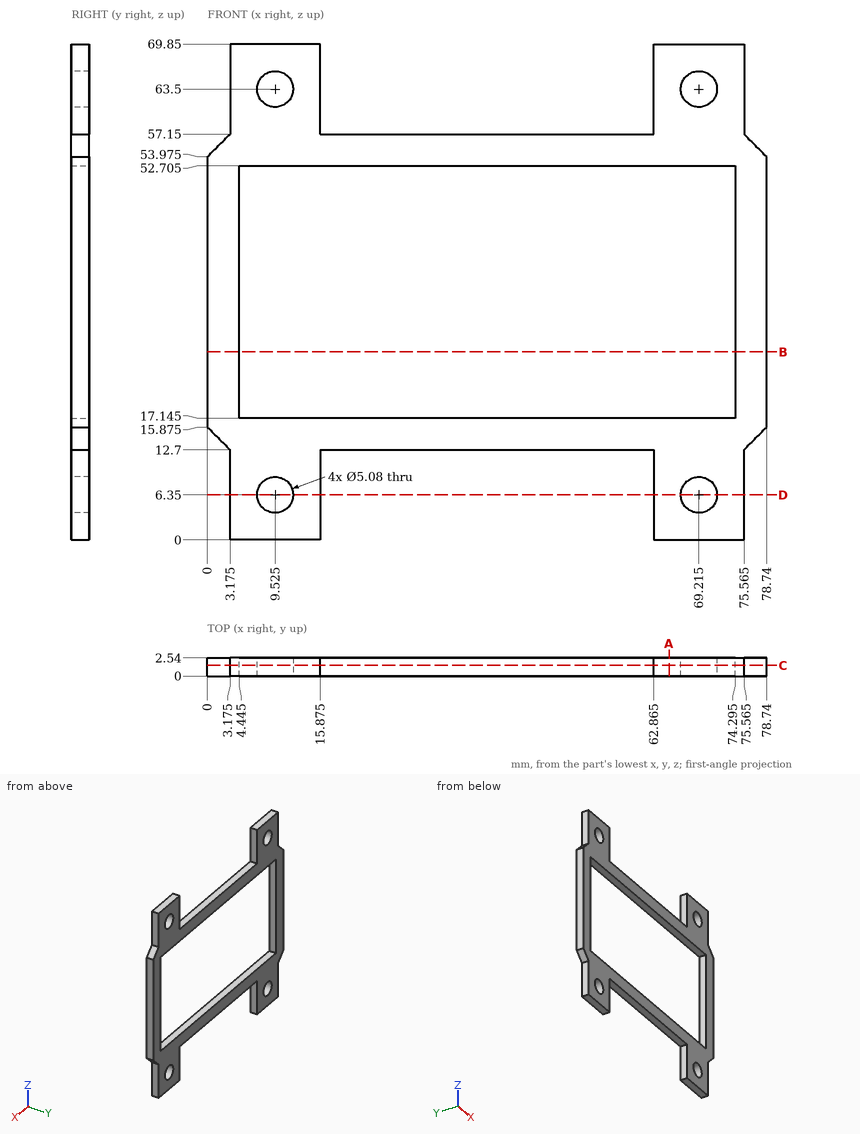
Geometry check sheet. Reference: drawing and pictorial views, mm from the part's lowest x, y, z. Round coordinates to 2 decimals unless told otherwise and drop trailing zeros. Write each loop counter-clockwise with the first axis right and the second up, starting at its lowest first coordinate (ties: lowest second). Pieces come first, ordered by that corner, then holes.
Item 1: Material ranges on line 1 along Z through (x, y) = (9.5, 0.4) (3 decimals); line 2 along Z through (x, y) = (30.5, 0.1) (3 decimals); line 3 along X through (y, z) = (1.8, 38.5) (3 decimals), recorded low to high.
Determined:
line 1: z = 0 to 3.81, 8.89 to 17.145, 52.705 to 60.96, 66.04 to 69.85
line 2: z = 12.7 to 17.145, 52.705 to 57.15
line 3: x = 0 to 4.445, 74.295 to 78.74
Item 2: Section check B-B (z = 26.5). Record the boundary of the cut face in (x, y) (3 decimals), plus the area to 3 significant figures.
Determined:
outline: (0, 0) - (4.445, 0) - (4.445, 2.54) - (0, 2.54) - close; (74.295, 0) - (78.74, 0) - (78.74, 2.54) - (74.295, 2.54) - close
area: 22.6 mm2
Item 3: Section check A-A (x = 65). Record the boundary of the cut face in (y, z) (3 decimals).
Determined:
outline: (0, 0) - (2.54, 0) - (2.54, 17.145) - (0, 17.145) - close; (0, 52.705) - (2.54, 52.705) - (2.54, 69.85) - (0, 69.85) - close
Item 4: Go/stop test with flat-tipped pins: pin 1 Ø0.8 at (y, z) = (0.5, 61.5) entering from +X (3 decimals); pin 2 Ø4 at (x, z) = (69.215, 63.5) entering from -Y; pin 3 Ø0.8 at (y, z) = (0.5, 8) entering from -X (3 decimals); pin 4 Ø1.3 at (x, y) = (22.5, 1.5) entering from +Z. Record where each tip stops, or that it passes through.
Determined:
pin 1: stops at x = 75.565
pin 2: passes through
pin 3: stops at x = 3.175
pin 4: stops at z = 57.15
Item 5: Section check D-D (z = 6.35). Record the boundary of the cut face in (x, y) (3 decimals).
Determined:
outline: (3.175, 0) - (6.985, 0) - (6.985, 2.54) - (3.175, 2.54) - close; (12.065, 0) - (15.875, 0) - (15.875, 2.54) - (12.065, 2.54) - close; (62.865, 0) - (66.675, 0) - (66.675, 2.54) - (62.865, 2.54) - close; (71.755, 0) - (75.565, 0) - (75.565, 2.54) - (71.755, 2.54) - close
Item 6: Section check C-C (y = 1.5). Record the boundary of the cut face in (x, z) (3 decimals).
Determined:
outline: (0, 15.875) - (3.175, 12.7) - (3.175, 0) - (15.875, 0) - (15.875, 12.7) - (62.865, 12.7) - (62.865, 0) - (75.565, 0) - (75.565, 12.7) - (78.74, 15.875) - (78.74, 53.975) - (75.565, 57.15) - (75.565, 69.85) - (62.865, 69.85) - (62.865, 57.15) - (15.875, 57.15) - (15.875, 69.85) - (3.175, 69.85) - (3.175, 57.15) - (0, 53.975) - close; hole (4.445, 17.145) - (74.295, 17.145) - (74.295, 52.705) - (4.445, 52.705) - close; hole circle Ø5.08 at (9.525, 6.35); hole circle Ø5.08 at (9.525, 63.5); hole circle Ø5.08 at (69.215, 6.35); hole circle Ø5.08 at (69.215, 63.5)
